Geometry check sheet. Reference: the model listing, model coordinates, mm. Round coordinates to 2 decimals unless told otherwise and drop trailing zeros. Order: outer loops, then holes, each group sorted by start corner. A loop starts at its lowest first (then second) coordinate and runs counter-clockwise, first axis right, second up. Notation, with made-up numbers: (22, -15.5) -> (43, -15.5) arc R17 ccw to (43, -4.5) -> close; hole circle Ø5 at (17, -18). An arc over 180 degrees is marked (long way). Use a Markdown table: item, result. Add a question column.
Item 1: Sectioned sample at A-A, the plane z = 7.25. State how many separate pieces and enclosed holes the cut face has, and give its area (3 significant figures).
Item 2: Sectioned sample at B-B, the plane y = 50. Record the cut outline in (x, z), and give its area (3 significant figures).
Item 3: Gauge pin test, flat ends, axial feed: pin 1 Ø1 at (x, z) = (8, 4) entering from -Y; pin 2 Ø2 at (x, z) = (6.5, 2) entering from +Y. Record the tip position at first contact, or that the pin passes through.
Item 4: Material ranges on probe 1 along Y at (x, z) = (6.25, 4.5); probe 2 along Y at (x, z) = (5.5, 7); probe 3 along X at (y, z) = (75, 5), recorded low to high. Write a range as [from, to].
from build123d import *

# Parameters (mm, degrees)
F0_W     = 12.5
F0_H     = 10
F1_DEPTH = 80
F2_R     = 2
F3_DEPTH = 10
F4_R     = 6.24999
F5_SIZE  = 1


# Not quite as in the source:
# - a fillet or chamfer is up to 0.001 mm smaller than in the source, because OpenCascade refuses the exact size


with BuildPart() as f1:
    # F0 (on Front) → F1 (new body)
    with BuildSketch(Plane.XZ):
        with Locations((6.25, 5)):
            Rectangle(F0_W, F0_H)
    extrude(amount=-F1_DEPTH)

    # F2 (on face) → F3 (cut, through all)
    with BuildSketch(Plane.XY.offset(10)):
        with Locations((6.25, 73.75)):
            Circle(F2_R)
        with Locations((6.25, 6.25)):
            Circle(F2_R)
    extrude(amount=-F3_DEPTH, mode=Mode.SUBTRACT)

    # F4 (radius 6.25 in the source; OpenCascade refuses exactly that, so slightly less here)
    f4_edges = [f1.edges().sort_by_distance(p)[0] for p in [
        (12.5, 0, 5),
        (0, 0, 5),
        (12.5, 80, 5),
        (0, 80, 5),
    ]]
    fillet(f4_edges, radius=F4_R)

    # F5
    f5_edges = [f1.edges().sort_by_distance(p)[0] for p in [
        (0, 40, 10),
        (0, 6.24999, 5),
        (0, 73.75001, 5),
        (0, 40, 0),
        (10.66942, 1.83058, 0),
        (6.25001, 0, 5),
        (12.5, 6.24999, 5),
        (10.66942, 1.83058, 10),
        (12.5, 40, 0),
        (12.5, 73.75001, 5),
        (12.5, 40, 10),
        (10.66942, 78.16942, 0),
        (6.25001, 80, 5),
        (10.66942, 78.16942, 10),
    ]]
    chamfer(f5_edges, length=F5_SIZE)


solid = f1.part
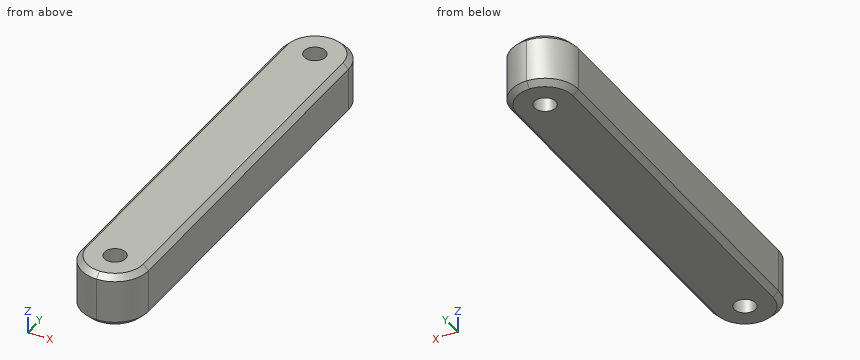
Found:
| question | item | result |
|---|---|---|
| 1 | separate pieces | 1 |
| 1 | enclosed holes | 2 |
| 1 | area | 941 mm2 |
| 2 | outline | (0, 1) -> (1, 0) -> (11.5, 0) -> (12.5, 1) -> (12.5, 9) -> (11.5, 10) -> (1, 10) -> (0, 9) -> close |
| 2 | area | 123 mm2 |
| 3 | pin 1 | stops at y = 0.13 |
| 3 | pin 2 | stops at y = 80 |
| 4 | probe 1 | y = [0, 4.25], [8.25, 71.75], [75.75, 80] |
| 4 | probe 2 | y = [0.05, 4.4], [8.1, 71.9], [75.6, 79.95] |
| 4 | probe 3 | x = [0.13, 4.69], [7.81, 12.37] |
